Check sheet for the drawn part. Datum: minimum x, y, z corner. Units: mm. Coordinates: 2 decimals unless noted, no trailing zeros. Write each loop counter-clockwise with the first axis right and the second up, starting at its lowest first coordinate (ties: lowest second). Pieces come first, ordered by that corner, then holes. Notation, with made-up numbers: (-21.75, 59) -> (-11.75, 59) arc R21 cw to (-11.75, 78) -> close; hole circle Ø7 at (88.5, 71). An arc over 180 degrees is marked (long way). Answer in a Markdown table with one row per item. Add a question column.
1. Depth check by flat-ended pin: P1, Ø1.5, axis at y = 2, z = 1.5, coming from the +X side; P2, Ø1.5, axis at x = 183.5, y = 2.5, coming from the -Z side; P3, Ø0.9, axis at x = 135.5, y = 1, coming from the +Z side. Enter the tip coordinate at first touch or a pass-through.
2. Scan lines: L1, parallel to X at y = 0.9, z = 41.5; L2, parallel to Z at x = 98, y = 1.15; L3, parallel to X at y = 0.75, z = 27. Record each from-to range of solid material in increasing order. Write a range as from..to.
3. Cross-section at A-A on x = 37. Record the cut outline in (y, z), and give its area (3 significant figures).
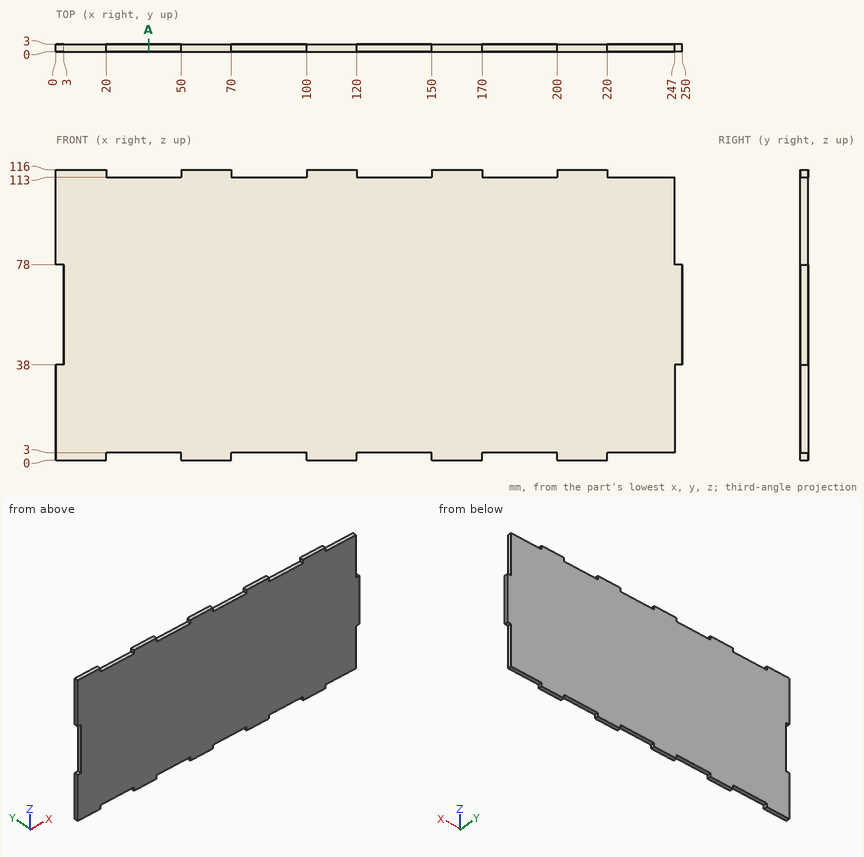
Results found:
| question | item | result |
|---|---|---|
| 1 | P1 | stops at x = 220 |
| 1 | P2 | stops at z = 3 |
| 1 | P3 | stops at z = 113 |
| 2 | L1 | x = 3..250 |
| 2 | L2 | z = 3..113 |
| 2 | L3 | x = 0..247 |
| 3 | outline | (0, 3) -> (3, 3) -> (3, 113) -> (0, 113) -> close |
| 3 | area | 330 mm^2 |
